Can you work these out from the drawing? Everything is in mm from the part's minimum corner. A direction names the side the tool comes from. Round coordinates to 2 decimals unless told otherwise and drop trailing zeros. Loops run counter-clockwise (first coordinate to the right, second up) from the corner with the lowest first, then second, coordinate; pieces in that order, holes last. Notation, with made-up numbers: (-24, -31.75) -> (17, -31.75) arc R32 cw to (17, -2.75) -> close; hole circle Ø11 at (6, 57.25). An arc over 180 degrees is marked (long way). Answer as a JSON object with one key per item and string values.
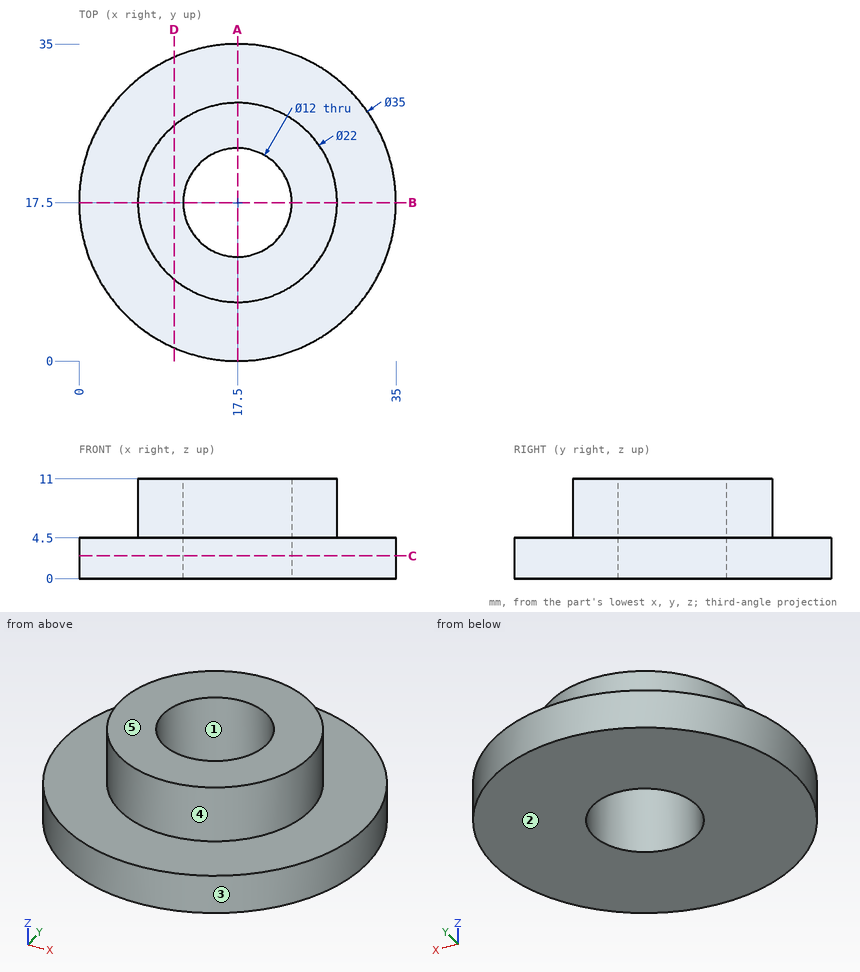
Q1. I want a section at D-D, the plane x = 10.5. Write out the boundary of the cut face in (y, z), then the cut area to 3 significant figures.
Determined:
{"outline": "(1.46, 0) -> (33.54, 0) -> (33.54, 4.5) -> (25.99, 4.5) -> (25.99, 11) -> (9.01, 11) -> (9.01, 4.5) -> (1.46, 4.5) -> close", "area": "255 mm²"}
Q2. On a 3-axis mill with a long thin cutter (end or side, diameter ignored), from which of +Z, -Z, +X, -X, +Y, -Y can I reach the whole of each face in a straight line? I mean the marked faces 4 and 5. Say none if no direction works.
Determined:
{"face 4": "+Z", "face 5": "+Z, +X, -X, +Y, -Y"}
Q3. We'd pull the mould along Y, two halves only. Please class the marked faces 1, 2 and 3: pulls with the +Y half, pulls with the -Y half, needs draft (parallel to the pull), parting line crosses it, or undercut.
Determined:
{"face 1": "undercut", "face 2": "needs draft", "face 3": "parting line crosses it"}
Q4. I want a section at A-A, the plane x = 17.5. Write out the boundary of the cut face in (y, z).
Determined:
{"outline": "(0, 0) -> (11.5, 0) -> (11.5, 11) -> (6.5, 11) -> (6.5, 4.5) -> (0, 4.5) -> close; (23.5, 0) -> (35, 0) -> (35, 4.5) -> (28.5, 4.5) -> (28.5, 11) -> (23.5, 11) -> close"}
Q5. If I drill on L1, parallel to Y at x = 17.5, z = 8.25; L2, parallel to Z at x = 9.5, y = 29; L3, parallel to Y at x = 19.5, z = 10.75, over which ranges is the centre line in solid material (lowest first)? Write a range as [from, to].
Determined:
{"L1": "[6.5, 11.5], [23.5, 28.5]", "L2": "[0, 4.5]", "L3": "[6.68, 11.84], [23.16, 28.32]"}
Q6. I want a section at C-C, the plane z = 2.5. Write out the boundary of the cut face in (x, y), then the cut area to 3 significant figures.
Determined:
{"outline": "circle Ø35 at (17.5, 17.5); hole circle Ø12 at (17.5, 17.5)", "area": "849 mm²"}
Q7. I'm going to push flat-ended pins straight in: pin 1 (3 mm diameter, centred on x = 11.5, z = 1, fed in from +Y); pin 2 (4 mm diameter, centred on x = 7, z = 4, fed in from -Y); pin 3 (10 mm diameter, centred on x = 15, y = 21, fed in from +Z); pin 4 (5 mm diameter, centred on y = 14.5, z = 2, fed in from +X). Where does each tip first touch, or does it pass through?
Determined:
{"pin 1": "y = 34.41", "pin 2": "y = 2.2", "pin 3": "z = 11", "pin 4": "x = 34.99"}
